Geometry check sheet. Reference: the model listing, model coordinates, mm. Face numbers are marked on the shaded views. A direction names the side the tool comes from. Round coordinates to 2 decimals unless told otherwise and drop trailing zeros. Write each loop counter-clockwise with the first axis right and the second up, starting at its lowest first coordinate (ties: lowest second). Pieces come first, ordered by that corner, then holes. Notation, with made-up numbers: (-1.75, 41.25) -> (17.25, 41.25) arc R13 ccw to (17.25, 55.25) -> close; hole circle Ø3 at (12.25, 1). An arc over 180 degrees is marked (long way). Use a Markdown table: item, result.
```python
from build123d import *

# Parameters (mm, degrees)
SKETCH082_W     = 28
SKETCH082_H     = 6
SKETCH082_R     = 2.05
PAD047_DEPTH    = 20
SKETCH083_R     = 2.05
POCKET032_DEPTH = 7
SKETCH084_R     = 2
PAD048_DEPTH    = 2
FILLET022_R     = 1.99
CHAMFER027_SIZE = 0.6
CHAMFER028_SIZE = 0.2


with BuildPart() as part:
    # Sketch082 → Pad047 (new body)
    with BuildSketch(Plane.XY):
        with Locations((-4, 3)):
            Rectangle(SKETCH082_W, SKETCH082_H)
        with Locations((-7, 3)):
            Circle(SKETCH082_R, mode=Mode.SUBTRACT)
        with Locations((6, 3)):
            Circle(SKETCH082_R, mode=Mode.SUBTRACT)
    extrude(amount=PAD047_DEPTH)

    # Sketch083 (on Face2 of Pad047) → Pocket032 (cut)
    with BuildSketch(Plane(origin=(-18, 0, 0), x_dir=(0, -1, 0), z_dir=(-1, 0, 0))):
        with Locations((-3, 15)):
            Circle(SKETCH083_R)
    extrude(amount=-POCKET032_DEPTH, mode=Mode.SUBTRACT)

    # Sketch084 (on Face3 of Pocket032) → Pad048 (join)
    with BuildSketch(Plane(origin=(-18, 0, 0), x_dir=(0, -1, 0), z_dir=(-1, 0, 0))):
        with Locations((-3, 5)):
            Circle(SKETCH084_R)
    extrude(amount=PAD048_DEPTH)

    # Fillet022
    fillet022_edges = [part.edges().sort_by_distance(p)[0] for p in [
        (-20, 5, 5),
    ]]
    fillet(fillet022_edges, radius=FILLET022_R)

    # Chamfer027
    chamfer027_edges = [part.edges().sort_by_distance(p)[0] for p in [
        (10, 0, 10),
        (10, 6, 10),
        (-18, 0, 10),
        (-18, 6, 10),
    ]]
    chamfer(chamfer027_edges, length=CHAMFER027_SIZE)

    # Chamfer028
    chamfer028_edges = [part.edges().sort_by_distance(p)[0] for p in [
        (-9.05, 3, 20),
        (3.95, 3, 20),
        (-9.05, 3, 0),
        (3.95, 3, 0),
        (-18, 5.05, 15),
    ]]
    chamfer(chamfer028_edges, length=CHAMFER028_SIZE)


with BuildPart() as part_1:
    # Body039 placement: moved
    add(part.part.moved(Location((-2e-06, 0, 13.5))))


solid = part_1.part
```
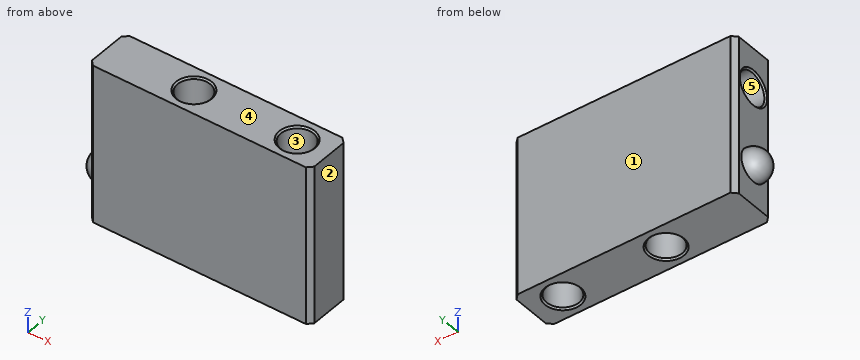
(1) Thickness scan on line 1 (X direction, y = 1.9, z = 18.75); line 2 (X direction, y = 1.3, z = 26); line 3 (Y direction, x = -7, z = 23.25). Record the ranges inside material, lowest first.
A:
| item | result |
|---|---|
| line 1 | x = -19.66 to -8.73, -5.27 to 4.27, 7.73 to 10 |
| line 2 | x = -18 to -8.15, -5.85 to 4.85, 7.15 to 10 |
| line 3 | y = 0 to 0.95, 5.05 to 6 |
(2) Section check A-A on z = 28.5. Record the cut outline in (x, y).
A:
| item | result |
|---|---|
| outline | (-18, 0.6) -> (-17.4, 0) -> (9.4, 0) -> (10, 0.6) -> (10, 5.4) -> (9.4, 6) -> (-17.4, 6) -> (-18, 5.4) -> (-18, 5.25) -> (-17.8, 5.05) -> (-11, 5.05) -> (-11, 0.95) -> (-17.8, 0.95) -> (-18, 0.75) -> close; hole circle Ø4.1 at (-7, 3); hole circle Ø4.1 at (6, 3) |
(3) Gauge pin test, flat end, axial feed: pin 1 Ø2 at (y, z) = (4, 29.5) entering from -X. Record the tip position at first contact, or that the pin passes through.
A:
| item | result |
|---|---|
| pin 1 | stops at x = -18 |
(4) Section check D-D on z = 16. Record the cut outline in (x, y).
A:
| item | result |
|---|---|
| outline | (-18, 0.6) -> (-17.4, 0) -> (9.4, 0) -> (10, 0.6) -> (10, 5.4) -> (9.4, 6) -> (-17.4, 6) -> (-18, 5.4) -> close; hole circle Ø4.1 at (-7, 3); hole circle Ø4.1 at (6, 3) |
(5) Section check B-B on x = -13. Record the cut outline in (y, z).
A:
| item | result |
|---|---|
| outline | (0, 13.5) -> (6, 13.5) -> (6, 33.5) -> (0, 33.5) -> close; hole circle Ø4.1 at (3, 28.5) |
(6) Section check C-C on y = 2.1. State how many separate pieces and enclosed holes the cut face has, plus the area to 3 significant figures.
A:
| item | result |
|---|---|
| separate pieces | 3 |
| enclosed holes | 0 |
| area | 392 mm2 |
(7) Release check for a two-part mould opening along Y. For the marked faces 1, 2 and 3 record: +Y half, -Y half, draft (parallel to the pull), parting line (faces both ways), or undercut.
A:
| item | result |
|---|---|
| face 1 | +Y half |
| face 2 | draft |
| face 3 | undercut |
(8) Access from +Z, -Z, +X, -X, +Y, -Y to the whole of each face (thin tool, end or side, straight path). Record for the marked faces 4 and 5.
A:
| item | result |
|---|---|
| face 4 | +Z, +X, -X, +Y, -Y |
| face 5 | -X |
